CAD build for the part. Positions are in the model's coordinates, mm. Face numbers are marked on the shaded views. A direction names the side the tool comes from. Give positions to 0.01 mm unless a question says otherwise; leave off trailing zeros. Order: outer loops, then holes, each group sorted by start corner. A loop starts at its lowest first (then second) coordinate and runs counter-clockwise, first axis right, second up. Notation, with made-up numbers: M -2.75,-7 L 14.25,-7 A15 cw 14.25,3 Z; hole C -3.75,-20 d10. An arc over 180 degrees is marked long. Put each result on its own line as item: value. Start each with the question number.
1) Cut at B-B (z = 46). Write the cut outline in (x, y), and give its area (3 significant figures).
2) Pin check, flat tips, straight feed: pin 1 (16 mm diameter, centred on y = 38.5, z = 0, fed in from -X); pin 2 (16 mm diameter, centred on y = -30.5, z = 6.5, fed in from -X); pin 3 (16 mm diameter, centred on x = 20, y = -34, fed in from +Z). Stop position of each tip, or through.
3) Cut at A-A (x = 8.75). Write the cut outline in (y, z), and give its area (3 significant figures).
4) Two-plate mould, pull along X, no slides. Class the marked faces 5, 6 and 7: released by +X, released by -X, zero draft, split by the parting line, or undercut.
5) Drill centre lines: line 1 (Y direction, x = 0, z = -3); line 2 (Y direction, x = -50, z = 86); line 3 (Y direction, x = 8.75, z = 6.5). Where is each one in solid material? Low to high. Write a range as [from, to].
6) Tool access for the marked faces 1, 2, 3 and 4: list every direction of +Z, -Z, +X, -X, +Y, -Y with a clear straight run to the whole face (end or side of a thin tool).
7) Cut at C-C (x = 63). Write the cut outline in (y, z).
Autodesk Fusion 360 part; units mm, degrees
sketch "Sketch1" plane through (0, 0, 0) normal (0, 0, 1) x (1, 0, 0)
  line L0 (50, -24) -> (-50, -24)
  line L1 (-50, -24) -> (-50, 24)
  line L2 (-50, 24) -> (50, 24)
  line L3 (50, 24) -> (50, -24)
  line L4 (50, -24) -> (-50, 24) construction
  line L5 (-50, -24) -> (50, 24) construction
  dimension "d1" = 100
  dimension "d2" = 48
extrude "Extrude1" add sketch "Sketch1" along normal blind 30
sketch "Sketch2" plane through (0, -24, 0) normal (0, -1, 0) x (1, 0, 0)
  line L0 (-50, 0) -> (50, 0)
  line L1 (50, 0) -> (50, 30)
  line L2 (50, 30) -> (-50, 30)
  line L3 (-50, 30) -> (-50, 0)
  line L4 (50, 0) -> (75, 0)
  line L5 (75, 0) -> (75, 60)
  line L6 (75, 60) -> (50, 60)
  line L7 (50, 60) -> (50, 0)
  line L8 (75, 60) -> (115, 60)
  line L9 (115, 60) -> (115, 0)
  line L10 (115, 0) -> (75, 0)
  line L11 (75, 0) -> (75, 60)
  line L12 (50, 60) -> (37.5, 30)
  circle A0 centre (-50, 60) radius 30
  circle A1 centre (-50, 60) radius 20
  line L13 (-15, 0) -> (33, 0)
  line L14 (33, 0) -> (33, 15)
  line L15 (33, 15) -> (-15, 15)
  line L16 (-15, 15) -> (-15, 0)
  line L17 (-50, 60) -> (-50, 70)
  line L18 (-50, 70) -> (-120, 70)
  line L19 (-120, 70) -> (-120, 67.5)
  line L20 (-120, 67.5) -> (-50, 52.5)
  line L21 (-50, 52.5) -> (-50, 60)
  line L22 (-50, 90) -> (-85, 90)
  line L23 (-85, 90) -> (-85, 70)
  line L24 (-85, 70) -> (-50, 70)
  line L25 (-50, 70) -> (-50, 90)
  line L26 (-20, 60) -> (-20, 30)
  dimension "d5" = 25
  dimension "d6" = 60
  dimension "d7" = 40
  dimension "d8" = 60
  dimension "d9" = 40
  dimension "d10" = 48
  dimension "d11" = 15
  dimension "d12" = 10
  dimension "d13" = 70
  dimension "d14" = 7.5
  dimension "d15" = 35
  dimension "d16" = 12.5
extrude "Extrude2" add sketch "Sketch2" against normal blind 48 contours L2 A0 L26 | A0 A1 L20 L25 | A0 L18 L19 L20 L24 | A0 A1 L18 L20 L24 | L1 L4 L5 L6 L7 L11 | L2 L7 L12 | A0 A1 L18 L24 L25
extrude "Extrude3" add sketch "Sketch2" against normal blind 20 from surface at -14 contours L5 L8 L9 L10 L11
extrude "Extrude4" add sketch "Sketch2" against normal blind 30 from surface at -10 contours A0 L18 L22 L23 L24
extrude "Extrude5" add sketch "Sketch2" along normal blind 20 contours L0 L13 L14 L15 L16
sketch "Sketch3" plane through (0, 0, 15) normal (0, 0, 1) x (-1, 0, 0)
  line L0 (-33, 24) -> (15, 24)
  line L1 (15, 24) -> (15, 44)
  line L2 (15, 44) -> (-33, 44)
  line L3 (-33, 44) -> (-33, 24)
  line L4 (-33, 24) -> (-3.4619, 53.5381)
  line L5 (-33, 24) -> (8.7732, 24) construction
  circle A0 centre (0, 35) radius 3.75
  dimension "d27" = 45
  dimension "d28" = 7.5
  dimension "d29" = 15
extrude "Extrude6" cut sketch "Sketch3" against normal blind 40 contours L2 L3 L4 | A0
mirror "Mirror1" about plane through (0, 0, 0) normal (0, 0, -1) of "Extrude5", "Extrude6"
mirror "Mirror2" about plane through (0, 0, 0) normal (0, 1, 0) of "Extrude5", "Mirror1"
hole "Hole1" at (-50, 1, 90) direction (0, 0, -1) diameter 7.5 depth 30 tip angle 180
hole "Hole2" at (8.75, 0, 30) direction (0, 0, -1) diameter 20 depth 60 tip angle 180 counterbore diameter 36 counterbore depth 2.5
fillet "Fillet1" radius 12.5 1 edges at (-20, 0, 30)
fillet "Fillet2" radius 2.5 6 edges at (75, -10, 30) (75, 10, 30) (75, 24, 30) (115, 10, 30) (115, -10, 30) (75, -24, 30)
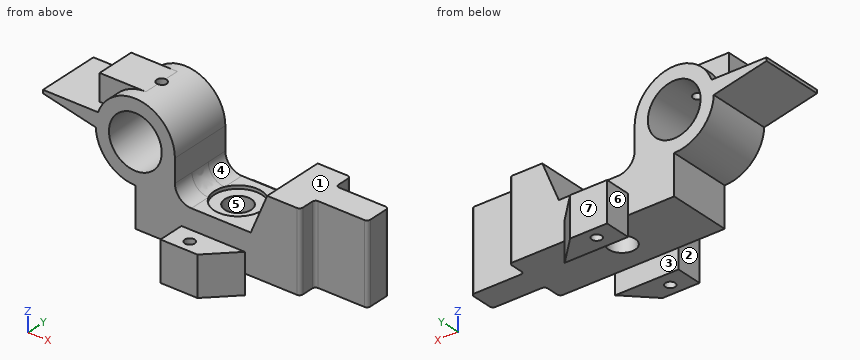
Solution:
1. outline: M -76.53,-24 L -64.28,-24 L -64.28,24 L -76.53,24 Z; M -35.72,-24 L -20,-24 L -20,24 L -35.72,24 Z; M 44.17,-24 L 72.5,-24 A2.5 ccw 75,-21.5 L 75,-12.5 A2.5 cw 77.5,-10 L 112.5,-10 A2.5 ccw 115,-7.5 L 115,7.5 A2.5 ccw 112.5,10 L 77.5,10 A2.5 cw 75,12.5 L 75,21.5 A2.5 ccw 72.5,24 L 44.17,24 Z
1. area: 3,620 mm²
2. pin 1: x = -15
2. pin 2: x = -50
2. pin 3: z = 15
3. outline: M -44,-15 L -24,-15 L -24,0 L -10,0 L -10,27.5 L -18,27.5 L -18,30 L -24,30 L -24,15 L -44,15 Z; M 10,0 L 24,0 L 24,-15 L 44,-15 L 44,15 L 24,15 L 24,30 L 18,30 L 18,27.5 L 10,27.5 Z
3. area: 2,000 mm²
4. face 5: undercut
4. face 6: released by -X
4. face 7: zero draft
5. line 1: [-44, -38.75], [-31.25, -24], [24, 31.25], [38.75, 44]
5. line 2: [-24, -2.75], [4.75, 24]
5. line 3: [-44, -10], [10, 44]
6. face 1: +Z, +X, +Y, -Y
6. face 2: +Z, -Z, -X, -Y
6. face 3: -Z, +X, -X
6. face 4: +Z, +Y, -Y
7. outline: M -24,0 L 24,0 L 24,60 L -24,60 Z
